Work out the finished part from the listing and answer in its coordinate system (mm). A direction names the side the tool comes from. Round coordinates to 2 decimals unless told otherwise and drop trailing zeros. Write each loop counter-clockwise with the first axis right and the second up, starting at its lowest first coordinate (ties: lowest second). Pieces come first, ordered by that corner, then holes. Notation, with made-up numbers: M -10.75,37.25 L 34.25,37.25 A25 ccw 34.25,56.25 Z; hole C 89.5,21 d3. An arc over 180 degrees is marked long. Answer in a Markdown table with one row per item.
```python
from build123d import *

# Parameters (mm, degrees)
SKETCH27_R          = 4
SKETCH27_R_2        = 2.5
SKETCH27_R_3        = 1.5
BOSS_EXTRUDE1_DEPTH = 6
SKETCH47_R          = 4.99
CUT_EXTRUDE8_DEPTH  = 3
SKETCH49_W          = 20
SKETCH49_H          = 6
CUT_EXTRUDE11_DEPTH = 3
CUT_EXTRUDE13_REACH = 97.747
SKETCH51_R          = 1.5
FILLET3_R           = 2
CHAMFER1_SIZE       = 1.5
FILLET5_START       = -1
FILLET5_DEPTH       = 4
SKETCH52_R          = 3
CUT_EXTRUDE14_DEPTH = 3
SKETCH53_R          = 1.5
CUT_EXTRUDE15_DEPTH = 3


with BuildPart() as part:
    # Sketch27 → Boss-Extrude1 (new body)
    with BuildSketch(Plane(origin=(0, 0, 0), x_dir=(0, 0, -1), z_dir=(1, 0, 0))):
        with BuildLine():
            Line((9, 50), (8.635545685, 50))
            ThreePointArc((8.635545685, 50), (11.67935283, 51.033233299), (13.465174817, 53.705904774))
            Line((13.465174817, 53.705904774), (16.829334589, 66.261119968))
            ThreePointArc((16.829334589, 66.261119968), (21.850788561, 69.160257771), (24.749926364, 64.138803798))
            ThreePointArc((24.749926364, 64.138803798), (27.861196202, 58.749926364), (33.250073636, 61.861196202))
            ThreePointArc((33.250073636, 61.861196202), (38.271527608, 64.760334004), (41.170665411, 59.738880032))
            Line((41.170665411, 59.738880032), (40.247638104, 56.294095226))
            ThreePointArc((40.247638104, 56.294095226), (41.110500534, 51.956192855), (45.077267236, 50))
            Line((45.077267236, 50), (66, 50))
            Line((66, 50), (66, 45))
            Line((66, 45), (51.734508099, 36))
            Line((51.734508099, 36), (43.997036047, 36))
            Line((43.997036047, 36), (40.577848346, 26.605858997))
            ThreePointArc((40.577848346, 26.605858997), (38.015035054, 23.26593569), (34, 22))
            Line((34, 22), (27, 22))
            ThreePointArc((27, 22), (21.089704308, 23.722694096), (17.030614343, 28.351199121))
            Line((17.030614343, 28.351199121), (14.396535233, 34))
            Line((14.396535233, 34), (9, 34))
            ThreePointArc((9, 34), (1, 42), (9, 50))
        make_face()
        with Locations((9, 42)):
            Circle(SKETCH27_R, mode=Mode.SUBTRACT)
        with Locations((50, 42)):
            Circle(SKETCH27_R_2, mode=Mode.SUBTRACT)
        with Locations((37.210369523, 60.800038117)):
            Circle(SKETCH27_R_3, mode=Mode.SUBTRACT)
        with Locations((20.789630477, 65.199961883)):
            Circle(SKETCH27_R_3, mode=Mode.SUBTRACT)
        with BuildLine():
            Line((29, 44), (28, 44))
            ThreePointArc((28, 44), (20.928932188, 41.071067812), (18, 34))
            Line((18, 34), (18, 33))
            ThreePointArc((18, 33), (20.636038969, 26.636038969), (27, 24))
            Line((27, 24), (34, 24))
            ThreePointArc((34, 24), (37.535533906, 25.464466094), (39, 29))
            Line((39, 29), (39, 34))
            ThreePointArc((39, 34), (36.071067812, 41.071067812), (29, 44))
        make_face(mode=Mode.SUBTRACT)
    extrude(amount=BOSS_EXTRUDE1_DEPTH)

    # Sketch47 → Cut-Extrude8 (cut)
    with BuildSketch(Plane.ZY):
        with Locations((-9, 42)):
            Circle(SKETCH47_R)
    extrude(amount=-CUT_EXTRUDE8_DEPTH, mode=Mode.SUBTRACT)

    # Sketch49 → Cut-Extrude11 (cut)
    with BuildSketch(Plane.ZY):
        with Locations((-30, 47)):
            Rectangle(SKETCH49_W, SKETCH49_H)
    extrude(amount=-CUT_EXTRUDE11_DEPTH, mode=Mode.SUBTRACT)

    # Sketch51 → Cut-Extrude13 (cut, up to next)
    with BuildSketch(Plane.ZY.offset(-3), mode=Mode.PRIVATE) as cut_extrude13_sk1:
        with Locations((-37, 47)):
            Circle(SKETCH51_R)
    cut_extrude13_tool1 = extrude(cut_extrude13_sk1.sketch, amount=-CUT_EXTRUDE13_REACH, mode=Mode.PRIVATE) & part.part
    # Sketch51 → Cut-Extrude13 (cut, up to next)
    with BuildSketch(Plane.ZY.offset(-3), mode=Mode.PRIVATE) as cut_extrude13_sk2:
        with Locations((-23, 47)):
            Circle(SKETCH51_R)
    cut_extrude13_tool2 = extrude(cut_extrude13_sk2.sketch, amount=-CUT_EXTRUDE13_REACH, mode=Mode.PRIVATE) & part.part
    add(cut_extrude13_tool1.solids().sort_by_distance((3, 47, -37))[0], mode=Mode.SUBTRACT)
    add(cut_extrude13_tool2.solids().sort_by_distance((3, 47, -23))[0], mode=Mode.SUBTRACT)

    # Fillet3
    fillet3_edges = [part.edges().sort_by_distance(p)[0] for p in [
        (3, 50, -66),
        (3, 45, -66),
        (3, 36, -51.734508099),
        (3, 36, -43.997036047),
        (3, 34, -14.396535233),
    ]]
    fillet(fillet3_edges, radius=FILLET3_R)

    # Chamfer1
    chamfer1_edges = [part.edges().sort_by_distance(p)[0] for p in [
        (6, 47, -38.5),
        (6, 47, -24.5),
        (6, 60.800038117, -35.710369523),
        (6, 65.199961883, -19.289630477),
    ]]
    chamfer(chamfer1_edges, length=CHAMFER1_SIZE)

    # Fillet5: read off the stored shape, not the designer's step
    # Fillet5 outline → Fillet5 (cut)
    with BuildSketch(Plane.YZ.offset(FILLET5_START)):
        with BuildLine():
            Line((44, -28), (44, -23.527864045))
            ThreePointArc((44, -23.527864045), (43.609108945, -24.015814081), (43.047619048, -23.7408229))
            ThreePointArc((43.047619048, -23.7408229), (43.75900073, -25.817821098), (44, -28))
        make_face()
        with BuildLine():
            ThreePointArc((44, -29), (43.75900073, -31.182178902), (43.047619048, -33.2591771))
            ThreePointArc((43.047619048, -33.2591771), (43.609108945, -32.984185919), (44, -33.472135955))
            Line((44, -33.472135955), (44, -29))
        make_face()
    extrude(amount=FILLET5_DEPTH, mode=Mode.SUBTRACT)

    # Sketch52 → Cut-Extrude14 (cut)
    with BuildSketch(Plane.ZY):
        with Locations((-50, 42)):
            Circle(SKETCH52_R)
    extrude(amount=-CUT_EXTRUDE14_DEPTH, mode=Mode.SUBTRACT)

    # Sketch53 → Cut-Extrude15 (cut)
    with BuildSketch(Plane.ZY):
        with Locations((-39, 49)):
            Circle(SKETCH53_R)
        with Locations((-21, 49)):
            Circle(SKETCH53_R)
        with Locations((-21, 45)):
            Circle(SKETCH53_R)
        with Locations((-39, 45)):
            Circle(SKETCH53_R)
    extrude(amount=-CUT_EXTRUDE15_DEPTH, mode=Mode.SUBTRACT)


solid = part.part
```
1. The part is cut by section C-C (x = 0.75). Count the separate pieces of the cut face and the enclosed holes in it, plus the area to 3 significant figures.
Calculated:
| item | result |
|---|---|
| separate pieces | 1 |
| enclosed holes | 5 |
| area | 948 mm² |
2. Consider line 1 along Y through (x, z) = (4.2, -37); line 2 along Y through (x, z) = (1.85, -50); line 3 along Y through (x, z) = (2.9, -25.5). Determine where each line is inside the solid, lowest interval first. Write a range as from..to.
Calculated:
| item | result |
|---|---|
| line 1 | y = 22.68..25, 40..45.5, 48.5..59.31, 62.29..64.89 |
| line 2 | y = 36..39, 45..50 |
| line 3 | y = 22.1..24.13, 50..60.33 |
3. Determine the mould class of faces 1 (the flat face through (3, 22, -31)), 2 (the cylindrical face through (4.48, 41.04, -52.31)), 3 (the flat face through (6, 46, -31)), 4 (the cylindrical face through (2.958, 51.006, -11.643)) for opening direction Y: released by +Y, released by -Y, zero draft, split by the parting line, or undercut.
Calculated:
| item | result |
|---|---|
| face 1 | released by -Y |
| face 2 | undercut |
| face 3 | zero draft |
| face 4 | released by +Y |
4. A tool of negligible diameter and unlimited length cuts with its end or side. For faces 5 (the flat face through (3, 34, -11)), 6 (the flat face through (3, 36, -48)), 7 (the cylindrical face through (3, 25, -37)), from which of +Z, -Z, +X, -X, +Y, -Y can it reach the whole face along a straight path? Write none if from no direction.
Calculated:
| item | result |
|---|---|
| face 5 | +Z, +X, -X, -Y |
| face 6 | -Z, +X, -X, -Y |
| face 7 | +X, -X |
5. The part is cut by section B-B (y = 41). Determine the outline of the cut face in (x, z).
Calculated:
| item | result |
|---|---|
| outline | M 0,-59.66 L 6,-59.66 L 6,-52.29 L 3,-52.29 L 3,-52.83 L 0,-52.83 Z; M 0,-47.17 L 3,-47.17 L 3,-47.71 L 6,-47.71 L 6,-36.14 L 0,-36.14 Z; M 0,-20.86 L 6,-20.86 L 6,-12.87 L 3,-12.87 L 3,-13.89 L 0,-13.89 Z; M 0,-4.11 L 3,-4.11 L 3,-5.13 L 6,-5.13 L 6,-1.06 L 0,-1.06 Z |
6. Given pin 1 (1.5 mm diameter, centred on x = 3, y = 46.5, fed in from +Z); pin 2 (3 mm diameter, centred on x = 2, z = -52.5, fed in from +Y); pin 3 (0.9 mm diameter, centred on x = 1, y = 47, fed in from +Z), each flat-ended and moving along its own axis, determine where each tip first touches the part or whether it passes through.
Calculated:
| item | result |
|---|---|
| pin 1 | stops at z = -1.93 |
| pin 2 | stops at y = 50 |
| pin 3 | stops at z = -2.42 |
7. The part is cut by section A-A (z = -50). Determine the outline of the cut face in (x, y).
Calculated:
| item | result |
|---|---|
| outline | M 0,36 L 6,36 L 6,39.5 L 3,39.5 L 3,39 L 0,39 Z; M 0,45 L 3,45 L 3,44.5 L 6,44.5 L 6,50 L 0,50 Z |
